Autodesk Inventor part; units mm, degrees
ref_plane "YZ Plane" through (0, 0, 0) normal (1, 0, 0) x (0, 1, 0)
ref_plane "XZ Plane" through (0, 0, 0) normal (0, 1, 0) x (-1, 0, 0)
ref_plane "XY Plane" through (0, 0, 0) normal (0, 0, 1) x (1, 0, 0)
sketch "Sketch1" plane through (0, 0, 0) normal (0, 1, 0) x (-1, 0, 0)
  circle A0 centre (0, 0) radius 152.4
  circle A1 centre (0, 0) radius 165.1
  dimension "d0" = 304.8
  dimension "d1" = 330.2
extrude "Extrusion1" add sketch "Sketch1" along normal blind 152.4
sketch "Sketch2" plane through (0, 0, 0) normal (1, 0, 0) x (0, 1, 0)
  circle A0 centre (100.6077, 0) radius 25.4
  point P0 (0, 0)
  dimension "d4" = 50.8
extrude "Extrusion2" add sketch "Sketch2" along normal mid plane 889
sketch "Sketch4" plane through (0, 152.4, 0) normal (0, 1, 0) x (1, 0, 0)
  circle A0 centre (0, 0) radius 152.4
extrude "Extrusion4" cut sketch "Sketch4" against normal through all
sketch "Sketch5" plane through (0, 152.4, 0) normal (0, 1, 0) x (1, 0, 0)
  circle A0 centre (0, 0) radius 165.1
extrude "Extrusion5" add sketch "Sketch5" along normal blind 50.8 draft -50
sketch "Sketch6" plane through (0, 152.4, 0) normal (0, -1, 0) x (1, 0, 0)
  circle A0 centre (0, 0) radius 104.5589
  circle A1 centre (0, 0) radius 50.8
  dimension "d15" = 101.6
extrude "Extrusion6" add sketch "Sketch6" along normal blind 254 contours A1
sketch "Sketch7" plane through (0, -101.6, 0) normal (0, -1, 0) x (1, 0, 0)
  circle A0 centre (0, 0) radius 104.5589
  circle A1 centre (0, 0) radius 101.6
  dimension "d18" = 203.2
extrude "Extrusion7" add sketch "Sketch7" along normal blind 25.4 contours A1
ref_plane "Work Plane1" through (0, 0, 0) normal (0, 1, 0) x (1, 0, 0)
sketch "Sketch8" plane through (0, 0, 0) normal (0, 1, 0) x (1, 0, 0)
  circle A0 centre (0, 0) radius 101.6
  dimension "d22" = 203.2
extrude "Extrusion8" add sketch "Sketch8" along normal blind 25.4
ref_plane "Work Plane2" through (75.376, -18.8821, -44.9646) normal (1, 0, 0) x (0, 1, 0)
sketch "Sketch9" plane through (75.376, -18.8821, -44.9646) normal (1, 0, 0) x (0, 1, 0)
  circle A0 centre (-604.603, 44.9646) radius 12.7
  point P0 (18.8821, 44.9646)
  dimension "d25" = 25.4
extrude "Extrusion9" cut sketch "Sketch9" against normal through all
properties part number "capistan upper"
The model under review builds one solid part; all positions refer to its coordinate system, in mm. A direction names the side the tool comes from. Round coordinates to 2 decimals unless told otherwise and drop trailing zeros. Order: outer loops, then holes, each group sorted by start corner. A loop starts at its lowest first (then second) coordinate and runs counter-clockwise, first axis right, second up. Notation, with made-up numbers: (-32.75, 58) -> (1.25, 58) arc R8 ccw to (1.25, 73) -> close; hole circle Ø1 at (11, -37). An arc over 180 degrees is marked (long way). Write item = value, one per line. Start each with the question number.
Item 1: Consider section A-A on x = 0. Write out the cut boundary in (y, z).
Item 2: For line 1 along Z through (x, y) = (0, 35); line 2 along X through (y, z) = (86, 0); line 3 along Y through (x, z) = (-60, 57), list the stretches that pass through material, from the lowest coordinate up.
Item 3: Consider section D-D on x = -265. Write out the cut boundary in (y, z), plus the area to 3 significant figures.
Item 4: Clearance check with flat-ended pins moving along their axes: pin 1 Ø12 at (x, z) = (-69.5, 105.5) entering from +Y; pin 2 Ø6 at (y, z) = (163, 58.5) entering from -X; pin 3 Ø5 at (y, z) = (10, 114.5) entering from +X; pin 4 Ø5 at (y, z) = (-38.5, 55.5) entering from +X. State where each tip first meets the part, or that it passes through.
Item 5: Mouldability with a two-part tool opening along Z and no side actions: class faces 6 (the face through (-22.025, 12.522, -99.184)), 7 (the face through (-150.784, 77.267, 22.132)), 8 (the face through (444.5, 100, 0)), 9 (the face through (50, 200.02, -96.12)) as released by +Z, released by -Z, zero draft, split by the parting line, or undercut.
Item 6: Consider section C-C on y = -36.5. Write out the cut boundary in (x, z), plus the area to 3 significant figures.
Item 7: For faces 1 (the face through (-22.025, -114.122, 99.184)), 2 (the face through (-301.847, 124.835, 7.629)), 3 (the face through (-1, -127, 1)), 4 (the face through (21, -101.6, 47)), 5 (the face through (301.847, 124.835, -7.629)), list the 3-axis set-ups (+Z, -Z, +X, -X, +Y, -Y) from which the entire face can be reached by the end or side of a thin tool; tool diameter is ignored.
Conclusion:
q1.outline = (-127, -101.6) -> (-101.6, -101.6) -> (-101.6, -50.8) -> (0, -50.8) -> (0, -101.6) -> (25.4, -101.6) -> (25.4, -50.8) -> (152.4, -50.8) -> (152.4, -152.4) -> (0, -152.4) -> (0, -165.1) -> (152.4, -165.1) -> (203.2, -104.56) -> (203.2, 104.56) -> (152.4, 165.1) -> (0, 165.1) -> (0, 152.4) -> (152.4, 152.4) -> (152.4, 50.8) -> (25.4, 50.8) -> (25.4, 101.6) -> (0, 101.6) -> (0, 50.8) -> (-101.6, 50.8) -> (-101.6, 101.6) -> (-127, 101.6) -> close
q2.line_1 = -165.1 to -152.4, -50.8 to 50.8, 152.4 to 165.1
q2.line_2 = -444.5 to -152.4, -50.8 to 50.8, 152.4 to 444.5
q2.line_3 = -127 to -101.6, 0 to 25.4, 152.4 to 203.2
q3.outline = circle Ø50.8 at (100.61, 0)
q3.area = 2,030 mm2
q4.pin_1 = 189.96
q4.pin_2 = -144.85
q4.pin_3 = 121.3
q4.pin_4 = through
q5.face_6 = undercut
q5.face_7 = undercut
q5.face_8 = zero draft
q5.face_9 = split by the parting line
q6.outline = circle Ø101.6 at (0, 0)
q6.area = 8,110 mm2
q7.face_1 = -Y
q7.face_2 = -X
q7.face_3 = +Z, -Z, +X, -X, -Y
q7.face_4 = none
q7.face_5 = +X
